from build123d import *

# Parameters (mm, degrees)
CROQUIS1_W              = 50.8
CROQUIS1_H              = 76.2
SALIENTE_EXTRUIR1_DEPTH = 18
CROQUIS2_W              = 50.8
CROQUIS2_H              = 76.2
CROQUIS2_W_2            = 46.12
CROQUIS2_H_2            = 71.52
CROQUIS2_W_3            = 38.8
CROQUIS2_H_3            = 64.2
CORTAR_EXTRUIR1_DEPTH   = 15
CORTAR_EXTRUIR8_DEPTH   = 15
SALIENTE_EXTRUIR3_DEPTH = 41.5
CORTAR_EXTRUIR9_DEPTH   = 51.5
CORTAR_EXTRUIR10_DEPTH  = 51.5
SALIENTE_EXTRUIR4_DEPTH = 16
CORTAR_EXTRUIR11_DEPTH  = 16.5
REDONDEO3_R             = 2
REDONDEO4_R             = 1
CROQUIS15_W             = 48.12
CROQUIS15_H             = 10
CORTAR_EXTRUIR12_DEPTH  = 15
CROQUIS16_W             = 8
CROQUIS16_H             = 1.5
CORTAR_EXTRUIR13_DEPTH  = 2
CROQUIS17_R             = 4
CROQUIS17_R_2           = 3
CORTAR_EXTRUIR14_DEPTH  = 10


with BuildPart() as part:
    # Croquis1 → Saliente-Extruir1 (new body)
    with BuildSketch(Plane.XY):
        Rectangle(CROQUIS1_W, CROQUIS1_H)
    extrude(amount=SALIENTE_EXTRUIR1_DEPTH)

    # Croquis2 → Cortar-Extruir1 (cut)
    # profile 1 of 2: a face of its own
    with BuildSketch(Plane.XY.offset(18)):
        Rectangle(CROQUIS2_W, CROQUIS2_H)
        Rectangle(CROQUIS2_W_2, CROQUIS2_H_2, mode=Mode.SUBTRACT)
    # profile 2 of 2: a face of its own
    with BuildSketch(Plane.XY.offset(18)):
        Rectangle(CROQUIS2_W_3, CROQUIS2_H_3)
    extrude(amount=-CORTAR_EXTRUIR1_DEPTH, mode=Mode.SUBTRACT)

    # Croquis6 → Cortar-Extruir8 (cut)
    with BuildSketch(Plane.XY.offset(18)):
        Polygon((-23.06, 35.76), (-8.06, 35.76), (-8.06, 32.1), (-19.4, 32.1), (-19.4, 20.76), (-23.06, 20.76), align=None)
        Polygon((23.06, 35.76), (8.06, 35.76), (8.06, 32.1), (19.4, 32.1), (19.4, 20.76), (23.06, 20.76), align=None)
        Polygon((-23.06, -35.76), (-23.06, -20.76), (-19.4, -20.76), (-19.4, -32.1), (-8.06, -32.1), (-8.06, -35.76), align=None)
        Polygon((23.06, -35.76), (8.06, -35.76), (8.06, -32.1), (19.4, -32.1), (19.4, -20.76), (23.06, -20.76), align=None)
    extrude(amount=-CORTAR_EXTRUIR8_DEPTH, mode=Mode.SUBTRACT)

    # Croquis10 → Saliente-Extruir3 (add)
    with BuildSketch(Plane(origin=(0, -20.76, 0), x_dir=(-1, 0, 0), z_dir=(0, -1, 0))):
        Polygon((23.06, -18), (24.06, -18), (23.06, -3), align=None)
        Polygon((-23.06, -18), (-24.06, -18), (-23.06, -3), align=None)
    extrude(amount=-SALIENTE_EXTRUIR3_DEPTH)

    # Croquis11 → Cortar-Extruir9 (cut)
    with BuildSketch(Plane.XZ.offset(20.76)):
        Polygon((-19.4, 18), (-21.56, 18), (-20.56, 3), (-19.4, 3), align=None)
    extrude(amount=-CORTAR_EXTRUIR9_DEPTH, mode=Mode.SUBTRACT)

    # Croquis12 → Cortar-Extruir10 (cut)
    with BuildSketch(Plane.XZ.offset(20.76)):
        Polygon((19.4, 18), (19.4, 3), (20.56, 3), (21.56, 18), align=None)
    extrude(amount=-CORTAR_EXTRUIR10_DEPTH, mode=Mode.SUBTRACT)

    # Croquis13 → Saliente-Extruir4 (add)
    with BuildSketch(Plane(origin=(8.06, 0, 0), x_dir=(0, 0, -1), z_dir=(1, 0, 0))):
        Polygon((-18, -35.76), (-18, -37.76), (-3, -35.76), align=None)
        Polygon((-18, 35.76), (-18, 37.76), (-3, 35.76), align=None)
    extrude(amount=-SALIENTE_EXTRUIR4_DEPTH)

    # Croquis14 → Cortar-Extruir11 (cut)
    with BuildSketch(Plane(origin=(8.06, 0, 0), x_dir=(0, 0, -1), z_dir=(1, 0, 0))):
        Polygon((-3, -32.1), (-18, -32.1), (-18, -35.26), (-3, -33.26), align=None)
        Polygon((-18, 32.1), (-18, 35.26), (-3, 33.26), (-3, 32.1), align=None)
    extrude(amount=-CORTAR_EXTRUIR11_DEPTH, mode=Mode.SUBTRACT)

    # Redondeo3
    redondeo3_edges = [part.edges().sort_by_distance(p)[0] for p in [
        (-25.4, 38.1, 1.5),
        (25.4, 38.1, 1.5),
        (25.4, -38.1, 1.5),
        (-25.4, -38.1, 1.5),
    ]]
    fillet(redondeo3_edges, radius=REDONDEO3_R)

    # Redondeo4
    redondeo4_edges = [part.edges().sort_by_distance(p)[0] for p in [
        (0, 38.1, 0),
        (-25.4, 0, 0),
        (25.4, 0, 0),
        (0, -38.1, 0),
        (24.814213562, -37.514213562, 0),
        (-24.814213562, -37.514213562, 0),
        (-24.814213562, 37.514213562, 0),
        (24.814213562, 37.514213562, 0),
    ]]
    fillet(redondeo4_edges, radius=REDONDEO4_R)

    # Croquis15 → Cortar-Extruir12 (cut)
    with BuildSketch(Plane.XY.offset(18)):
        with Locations((0, -0.01)):
            Rectangle(CROQUIS15_W, CROQUIS15_H)
    extrude(amount=-CORTAR_EXTRUIR12_DEPTH, mode=Mode.SUBTRACT)

    # Croquis16 → Cortar-Extruir13 (cut)
    with BuildSketch(Plane.XZ.offset(38.1)):
        with Locations((0, 2.25)):
            Rectangle(CROQUIS16_W, CROQUIS16_H)
    extrude(amount=-CORTAR_EXTRUIR13_DEPTH, mode=Mode.SUBTRACT)

    # Croquis17 → Cortar-Extruir14 (cut)
    with BuildSketch(Plane.XY.offset(3)):
        with Locations((10.4, 23.1)):
            Circle(CROQUIS17_R)
        with Locations((10.4, 14.1)):
            Circle(CROQUIS17_R_2)
    extrude(amount=-CORTAR_EXTRUIR14_DEPTH, mode=Mode.SUBTRACT)


solid = part.part
Geometry: final body of the model. Coordinates: model frame, mm. A direction names the side the tool comes from. Coordinates: 2 decimals unless noted, no trailing zeros. Order: outer loops, then holes, each group sorted by start corner. A loop starts at its lowest first (then second) coordinate and runs counter-clockwise, first axis right, second up. Notation, with made-up numbers: M -34,39.5 L 19,39.5 A38 cw 19,77.5 Z; hole C 83.25,-9 d4. An arc over 180 degrees is marked long. One line per question, with ' | ' between items. Start each with the question number.
Item 1: Cut plane D-D, the plane x = 5. Return the cut outline in (y, z).
Item 2: Cut plane B-B, the plane z = 17.25. Count the separate pieces of the cut face and the enclosed holes in it, then the cut area to 3 significant figures.
Item 3: Draft query along X for faces 4 (the flat face through (-7.94, -36.5, 12.3)), 5 (the flat face through (0.172, -36.774, 10.605)), 6 (the flat face through (21.053, 12.765, 10.395)). Return one class per face: released by +X, released by -X, zero draft, split by the parting line, or undercut.
Item 4: Cut plane A-A, the plane x = 10.4. Return the cut outline in (y, z).
Item 5: Cut plane C-C, the plane y = 14.1. Return the cut outline in (x, z), then the cut area to 3 significant figures.
Item 6: Pin query (flat end, axial travel): pin 1 Ø0.8 at (x, z) = (-23.5, 9) entering from +Y; pin 2 Ø10 at (y, z) = (-14, 7.5) entering from -X; pin 3 Ø1.2 at (x, z) = (-0.5, 2.5) entering from -Y; pin 4 Ø10 at (x, z) = (12.5, 11) entering from -Y. Return the tip coordinate at first contact, or that it passes through.
Item 7: Ray query, probe 1 along Y at (x, z) = (10.4, 1.75); probe 2 along Z at (x, y) = (2.5, 33); probe 3 along Y at (x, z) = (22, 8.5). Return the intervals inside material, ascending. Write a range as [from, to].
Item 8: Set-up query: faces 1 (the flat face through (22, -5.01, 11)), 2 (the flat face through (-22, -20.76, 10)), 3 (the flat face through (-22, 20.76, 11)). Return all of +Z, -Z, +X, -X, +Y, -Y with unobstructed straight access to the full face (end or side cutting, diameter ignored); none if empty.
A:
1) outline: M -38.1,1 A1 ccw -37.1,0 L 37.1,0 A1 ccw 38.1,1 L 38.1,3 L 35.76,3 L 37.76,18 L 35.26,18 L 33.26,3 L -33.26,3 L -35.26,18 L -37.76,18 L -35.76,3 L -38.1,3 Z
2) separate pieces: 6 | enclosed holes: 0 | area: 238 mm2
3) face 4: released by -X | face 5: zero draft | face 6: undercut
4) outline: M -38.1,1 A1 ccw -37.1,0 L 11.1,0 L 11.1,3 L -38.1,3 Z; M 17.1,0 L 19.1,0 L 19.1,3 L 17.1,3 Z; M 27.1,0 L 37.1,0 A1 ccw 38.1,1 L 38.1,3 L 27.1,3 Z
5) outline: M -25.4,1 A1 ccw -24.4,0 L 7.4,0 L 7.4,3 L -20.56,3 L -21.56,18 L -24.06,18 L -23.06,3 L -25.4,3 Z; M 13.4,0 L 24.4,0 A1 ccw 25.4,1 L 25.4,3 L 23.06,3 L 24.06,18 L 21.56,18 L 20.56,3 L 13.4,3 Z | area: 209 mm2
6) pin 1: stops at y = 20.74 | pin 2: stops at x = -25.4 | pin 3: stops at y = -36.1 | pin 4: stops at y = -37.13
7) probe 1: y = [-38.1, 11.1], [17.1, 19.1], [27.1, 38.1] | probe 2: z = [0, 3] | probe 3: y = [-20.76, -5.01], [4.99, 20.76]
8) face 1: +Z, +X, -X | face 2: +Z, +X, -X, -Y | face 3: +Z, +X, -X, +Y
